Model file for the job. Use its own axes, mm. Face numbers are marked on the shaded views. Coordinates: 2 decimals unless noted, no trailing zeros. Order: outer loops, then holes, each group sorted by start corner. A loop starts at its lowest first (then second) coordinate and runs counter-clockwise, first axis right, second up.
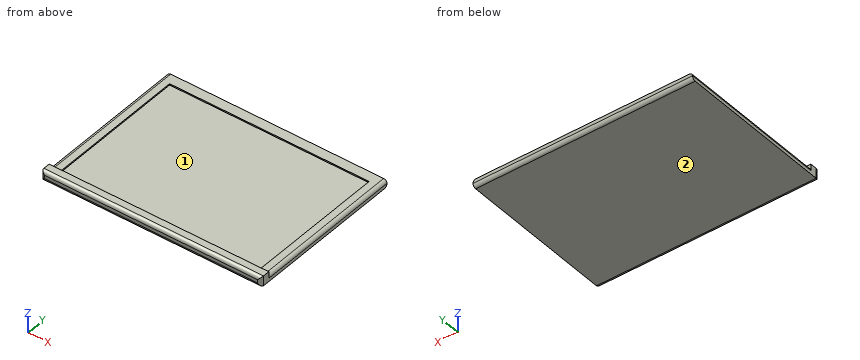
from build123d import *

# Parameters (mm, degrees)
F1_DEPTH = 10
F0_W     = 298
F0_H     = 211
F2_DEPTH = 8
F3_DEPTH = 15
F4_R     = 4.99999


# Not quite as in the source:
# - a fillet or chamfer is up to 0.001 mm smaller than in the source, because OpenCascade refuses the exact size


with BuildPart() as f1:
    # F0 (on Top) → F1 (new body)
    with BuildSketch(Plane.XY):
        Polygon((-149, -105.5), (-149, 105.5), (149, 105.5), (149, -105.5), (164, -105.5), (164, 120.5), (-164, 120.5), (-164, -105.5), align=None)
    extrude(amount=F1_DEPTH)

    # F0 (on Top) → F2 (join)
    with BuildSketch(Plane.XY):
        Rectangle(F0_W, F0_H)
    extrude(amount=F2_DEPTH)

    # F0 (on Top) → F3 (join)
    with BuildSketch(Plane.XY):
        Polygon((149, -105.5), (-149, -105.5), (-164, -105.5), (-164, -120.5), (164, -120.5), (164, -105.5), align=None)
    extrude(amount=F3_DEPTH)

    # F4 (radius 5 in the source; OpenCascade refuses exactly that, so slightly less here)
    f4_edges = [f1.edges().sort_by_distance(p)[0] for p in [
        (0, 120.5, 0),
        (-164, 7.5, 10),
        (164, 7.5, 10),
        (0, -120.5, 15),
        (164, -120.5, 7.5),
        (-164, -120.5, 7.5),
        (0, -120.5, 0),
    ]]
    fillet(f4_edges, radius=F4_R)


solid = f1.part
Q1. Drop flat-ended pins along their axis: P1, Ø1, axis at y = 84, z = 7, coming from the +X side; P2, Ø1, axis at y = 10, z = 9, coming from the +X side; P3, Ø1, axis at y = 67.5, z = 9, coming from the -X side. Give the stop position or say it passes through.
Established:
P1: stops at x = 163.77
P2: stops at x = 162.57
P3: stops at x = -162.57
Q2. Mould opens along X. For the marked faces 1 and 2 say: pulls with the +X half, pulls with the -X half, needs draft (parallel to the pull), parting line crosses it, or undercut.
Established:
face 1: undercut
face 2: needs draft
Q3. Probe line 1 (Y direction, x = 102.5, z = 9); line 2 (Z direction, x = 97.5, y = 90); line 3 (X direction, y = -76, z = 9.25). List the from-to ranges inside material, lowest first.
Established:
line 1: y = -120.5 to -105.5, 105.5 to 120.5
line 2: z = 0 to 8
line 3: x = -161.63 to -149, 149 to 161.63
Q4. Cut at A-A, the plane x = -47.5. List the corners of the cut face in (y, z).
Established:
outline: (-120.5, 5) arc R5 ccw to (-115.5, 0) - (115.5, 0) arc R5 ccw to (120.5, 5) - (120.5, 10) - (105.5, 10) - (105.5, 8) - (-105.5, 8) - (-105.5, 15) - (-115.5, 15) arc R5 ccw to (-120.5, 10) - close
Q5. Cut at B-B, the plane y = 13. List the corners of the cut face in (x, z).
Established:
outline: (-164, 0) - (164, 0) - (164, 5) arc R5 ccw to (159, 10) - (149, 10) - (149, 8) - (-149, 8) - (-149, 10) - (-159, 10) arc R5 ccw to (-164, 5) - close
